The model under review builds one solid part; all positions refer to its coordinate system, in mm. Face numbers are marked on the shaded views. A direction names the side the tool comes from. Coordinates: 2 decimals unless noted, no trailing zeros.
```python
from build123d import *

# Parameters (mm, degrees)
SKETCH2_R           = 145
SKETCH2_R_2         = 105
BOSS_EXTRUDE1_START = -50
SKETCH3_W           = 360
SKETCH3_H           = 360
SKETCH3_R           = 145
BOSS_EXTRUDE1_DEPTH = 50
FILLET1_R           = 20
SKETCH4_R           = 145
BOSS_EXTRUDE2_DEPTH = 50
SKETCH5_R           = 30
CUT_EXTRUDE1_DEPTH  = 10
SKETCH6_R           = 15
CUT_EXTRUDE2_DEPTH  = 86
CIRPATTERN1_COUNT   = 4
SKETCH9_R           = 30
CUT_EXTRUDE3_DEPTH  = 10
CUT_EXTRUDE4_REACH  = 848.699
SKETCH10_R          = 15
CIRPATTERN2_COUNT   = 4
CHAMFER1_SIZE       = 10


with BuildPart() as part:
    # Sweep-Thin1: sweep along a path in Sketch1
    with BuildLine(Plane.XY) as sweep_thin1_path:
        Line((0, 0), (-150, 0))
        ThreePointArc((-150, 0), (-333.847763109, 76.152236891), (-410, 260))
        Line((-410, 260), (-410, 410))
    # Sketch2 → Sweep-Thin1 (sweep)
    with BuildSketch(Plane(origin=(0, 0, 0), x_dir=(0, 0, -1), z_dir=(1, 0, 0))):
        Circle(SKETCH2_R)
        Circle(SKETCH2_R_2, mode=Mode.SUBTRACT)
    sweep(path=sweep_thin1_path.line)

    # Sketch3 → Boss-Extrude1 (add)
    with BuildSketch(Plane(origin=(0, 0, 0), x_dir=(0, 0, -1), z_dir=(1, 0, 0)).offset(BOSS_EXTRUDE1_START)):
        Rectangle(SKETCH3_W, SKETCH3_H)
        with Locations(Location((0, 0, 0), (0, 0, 270))):
            Circle(SKETCH3_R, mode=Mode.SUBTRACT)
    extrude(amount=BOSS_EXTRUDE1_DEPTH)

    # Fillet1
    fillet1_edges = [part.edges().sort_by_distance(p)[0] for p in [
        (-25, 180, -180),
        (-25, -180, -180),
        (-25, -180, 180),
        (-25, 180, 180),
    ]]
    fillet(fillet1_edges, radius=FILLET1_R)

    # Sketch4 → Boss-Extrude2 (add)
    with BuildSketch(Plane(origin=(0, 410, 0), x_dir=(1, 0, 0), z_dir=(0, 1, 0))):
        with BuildLine():
            Line((-570, 180), (-250, 180))
            ThreePointArc((-250, 180), (-235.857864376, 174.142135624), (-230, 160))
            Line((-230, 160), (-230, -160))
            ThreePointArc((-230, -160), (-235.857864376, -174.142135624), (-250, -180))
            Line((-250, -180), (-570, -180))
            ThreePointArc((-570, -180), (-584.142135624, -174.142135624), (-590, -160))
            Line((-590, -160), (-590, 160))
            ThreePointArc((-590, 160), (-584.142135624, 174.142135624), (-570, 180))
        make_face()
        with Locations(Location((-410, 0, 0), (0, 0, 270))):
            Circle(SKETCH4_R, mode=Mode.SUBTRACT)
    extrude(amount=-BOSS_EXTRUDE2_DEPTH)

    # Sketch5 → Cut-Extrude1 (cut)
    with BuildSketch(Plane(origin=(0, 0, 0), x_dir=(0, 0, -1), z_dir=(1, 0, 0))):
        with Locations((-130, 130)):
            Circle(SKETCH5_R)
    cut_extrude1 = extrude(amount=-CUT_EXTRUDE1_DEPTH, mode=Mode.SUBTRACT)

    # Sketch6 → Cut-Extrude2 (cut)
    with BuildSketch(Plane(origin=(-10, 0, 0), x_dir=(0, 0, -1), z_dir=(1, 0, 0))):
        with Locations((-130, 130)):
            Circle(SKETCH6_R)
    cut_extrude2 = extrude(amount=-CUT_EXTRUDE2_DEPTH, mode=Mode.SUBTRACT)

    # CirPattern1: Cut-Extrude1, Cut-Extrude2 ×4 about axis
    cirpattern1_axis = Axis((0, 0, 0), (1, 0, 0))
    add([cut_extrude1.rotate(cirpattern1_axis, i * 360 / CIRPATTERN1_COUNT) for i in range(1, CIRPATTERN1_COUNT)], mode=Mode.SUBTRACT)
    add([cut_extrude2.rotate(cirpattern1_axis, i * 360 / CIRPATTERN1_COUNT) for i in range(1, CIRPATTERN1_COUNT)], mode=Mode.SUBTRACT)

    # Sketch9 → Cut-Extrude3 (cut)
    with BuildSketch(Plane(origin=(0, 410, 0), x_dir=(1, 0, 0), z_dir=(0, 1, 0))):
        with Locations(Location((-540, 130, 0), (0, 0, 270))):
            Circle(SKETCH9_R)
    cut_extrude3 = extrude(amount=-CUT_EXTRUDE3_DEPTH, mode=Mode.SUBTRACT)

    # Sketch10 → Cut-Extrude4 (cut, up to next)
    with BuildSketch(Plane(origin=(0, 400, 0), x_dir=(1, 0, 0), z_dir=(0, 1, 0)), mode=Mode.PRIVATE) as cut_extrude4_sk1:
        with Locations(Location((-540, 130, 0), (0, 0, 270))):
            Circle(SKETCH10_R)
    cut_extrude4_tool1 = extrude(cut_extrude4_sk1.sketch, amount=-CUT_EXTRUDE4_REACH, mode=Mode.PRIVATE) & part.part
    cut_extrude4 = cut_extrude4_tool1.solids().sort_by_distance((-540, 400, -130))[0]
    add(cut_extrude4, mode=Mode.SUBTRACT)

    # CirPattern2: Cut-Extrude3, Cut-Extrude4 ×4 about axis
    cirpattern2_axis = Axis((-410, 0, 0), (0, 1, 0))
    add([cut_extrude3.rotate(cirpattern2_axis, i * 360 / CIRPATTERN2_COUNT) for i in range(1, CIRPATTERN2_COUNT)], mode=Mode.SUBTRACT)
    add([cut_extrude4.rotate(cirpattern2_axis, i * 360 / CIRPATTERN2_COUNT) for i in range(1, CIRPATTERN2_COUNT)], mode=Mode.SUBTRACT)

    # Chamfer1
    chamfer1_edges = [part.edges().sort_by_distance(p)[0] for p in [
        (0, 0, 105),
        (-410, 410, 105),
    ]]
    chamfer(chamfer1_edges, length=CHAMFER1_SIZE)


solid = part.part
```
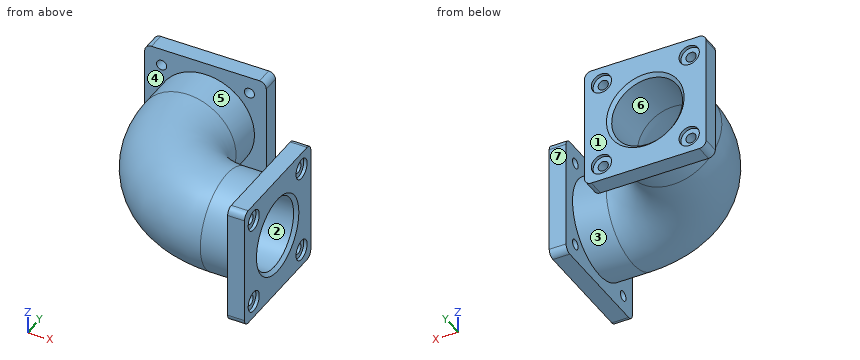
Item 1: Mouldability with a two-part tool opening along Y and no side actions: class the marked faces 1, 2, 3 and 4 as pulls with the +Y half, pulls with the -Y half, needs draft (parallel to the pull), parting line crosses it, or undercut.
Solved:
face 1: pulls with the +Y half
face 2: undercut
face 3: parting line crosses it
face 4: undercut
Item 2: For pin 1 (4 mm diameter, centred on x = -196.5, y = -69, fed in from +Z); pin 2 (6 mm diameter, centred on x = -100, z = -98, fed in from +Y); pin 3 (15 mm diameter, centred on x = -14, z = -2, fed in from +Y), all flat-tipped, find the tip position at first contact; note any pin that passes through.
Solved:
pin 1: stops at z = 126.84
pin 2: stops at y = 109.54
pin 3: stops at y = 180
Item 3: Machinability: for the marked faces 5, 6 and 7, which of the approach directions +Z, -Z, +X, -X, +Y, -Y give a long, thin tool a straight path to every point of the face, cutting with its end or side? Answer none if there is none.
Solved:
face 5: none
face 6: +Y
face 7: +Z, -Z, +X, +Y
Item 4: To check wall thickness, follow line 1 along Z through (x, y) = (-26.5, -130); line 2 along X through (y, z) = (402.75, 130); line 3 along X through (y, z) = (375, -130). State the ranges of each line that lie inside material, in increasing order.
Solved:
line 1: z = -180 to -145, -115 to 115, 145 to 180
line 2: x = -590 to -570, -510 to -310, -250 to -230
line 3: x = -590 to -555, -525 to -295, -265 to -230
Item 5: Take a section at A-A, the plane x = -280. Count the separate pieces of the cut face and the enclosed holes in it, plus the area to 3 significant figures.
Solved:
separate pieces: 3
enclosed holes: 1
area: 71,600 mm2
